Build history of the part. All positions in model axes, mm. A direction names the side the tool comes from. Round coordinates to 2 decimals unless told otherwise and drop trailing zeros. Loops run counter-clockwise (first coordinate to the right, second up) from the corner with the lowest first, then second, coordinate; pieces in that order, holes last. Notation, with made-up numbers: (-1, 26.25) - (19, 26.25) arc R10 cw to (19, 44.25) - close; hole circle Ø8 at (-38, 10). An arc over 180 degrees is marked (long way). Answer as CSV lines item,"result". Start each with the question number.
```python
from build123d import *

# Parameters (mm, degrees)
SKETCH_R      = 54
SKETCH_R_2    = 32
SKETCH_R_3    = 2.5
PAD_DEPTH     = 3
SKETCH001_R   = 37.5
SKETCH001_R_2 = 32.5
PAD001_DEPTH  = 4
SKETCH002_R   = 42
SKETCH002_R_2 = 37.5
PAD002_DEPTH  = 18
SKETCH003_R   = 48
SKETCH003_R_2 = 42
PAD003_DEPTH  = 5
SKETCH004_R   = 32
SKETCH004_R_2 = 5.25
POCKET_DEPTH  = 18.001
CHAMFER_SIZE  = 1


with BuildPart() as part:
    # Sketch → Pad (new body)
    with BuildSketch(Plane.XY):
        Circle(SKETCH_R)
        Circle(SKETCH_R_2, mode=Mode.SUBTRACT)
        with Locations((31.496593, 37.536178)):
            Circle(SKETCH_R_3, mode=Mode.SUBTRACT)
        with Locations((48.25558, 8.508761)):
            Circle(SKETCH_R_3, mode=Mode.SUBTRACT)
        with Locations((42.435245, -24.5)):
            Circle(SKETCH_R_3, mode=Mode.SUBTRACT)
        with Locations((16.758987, -46.044938)):
            Circle(SKETCH_R_3, mode=Mode.SUBTRACT)
        with Locations((-16.758987, -46.044938)):
            Circle(SKETCH_R_3, mode=Mode.SUBTRACT)
        with Locations((-42.435245, -24.5)):
            Circle(SKETCH_R_3, mode=Mode.SUBTRACT)
        with Locations((-48.25558, 8.508761)):
            Circle(SKETCH_R_3, mode=Mode.SUBTRACT)
        with Locations((-31.496593, 37.536178)):
            Circle(SKETCH_R_3, mode=Mode.SUBTRACT)
        with Locations((0, 49)):
            Circle(SKETCH_R_3, mode=Mode.SUBTRACT)
    extrude(amount=PAD_DEPTH)

    # Sketch001 (on Face13 of Pad) → Pad001 (join)
    with BuildSketch(Plane.XY.offset(3)):
        Circle(SKETCH001_R)
        Circle(SKETCH001_R_2, mode=Mode.SUBTRACT)
    extrude(amount=PAD001_DEPTH)

    # Sketch002 (on Face3 of Pad001) → Pad002 (join)
    with BuildSketch(Plane.XY.offset(3)):
        Circle(SKETCH002_R)
        Circle(SKETCH002_R_2, mode=Mode.SUBTRACT)
    extrude(amount=PAD002_DEPTH)

    # Sketch003 (on Face3 of Pad002) → Pad003 (join)
    with BuildSketch(Plane.XY.offset(3)):
        Circle(SKETCH003_R)
        Circle(SKETCH003_R_2, mode=Mode.SUBTRACT)
    extrude(amount=PAD003_DEPTH)

    # Sketch004 → Pocket (cut, through all)
    with BuildSketch(Plane.XY.offset(3)):
        Circle(SKETCH004_R)
        with Locations((31.496593, 37.536178)):
            Circle(SKETCH004_R_2)
        with Locations((48.25558, 8.508761)):
            Circle(SKETCH004_R_2)
        with Locations((42.435245, -24.5)):
            Circle(SKETCH004_R_2)
        with Locations((16.758987, -46.044938)):
            Circle(SKETCH004_R_2)
        with Locations((-16.758987, -46.044938)):
            Circle(SKETCH004_R_2)
        with Locations((-42.435245, -24.5)):
            Circle(SKETCH004_R_2)
        with Locations((-48.25558, 8.508761)):
            Circle(SKETCH004_R_2)
        with Locations((-31.496593, 37.536178)):
            Circle(SKETCH004_R_2)
        with Locations((0, 49)):
            Circle(SKETCH004_R_2)
    extrude(amount=POCKET_DEPTH, mode=Mode.SUBTRACT)

    # Chamfer
    chamfer_edges = [part.edges().sort_by_distance(p)[0] for p in [
        (-37.5, 0, 21),
        (-42, 0, 21),
    ]]
    chamfer(chamfer_edges, length=CHAMFER_SIZE)


solid = part.part
```
Q1. Pin check, flat tips, straight feed: pin 1 Ø5 at (x, y) = (-33, 3.5) entering from -Z; pin 2 Ø2 at (x, y) = (32, 34.5) entering from +Z; pin 3 Ø1.5 at (x, z) = (-19.5, 4.5) entering from +Y; pin 4 Ø8 at (y, z) = (18.5, 17.5) entering from +X. Stop position of each tip, or through.
Q2. Wall check: probe 1 along Y at (x, z) = (0, 16); probe 2 along Z at (x, y) = (-40, 33); probe 3 along Z at (x, y) = (-15, -31). Give the ranges that are in metal, low to high. Write a range as [from, to].
Q3. Band-saw the part on B-B, the plane z = 4.75. List the corners of the cut face in (x, y), then the cut area to 3 significant figures.
Q4. Tool access for faces 4 (the cylindrical face through (31, 9.76, 4.97)), 5 (the cylindrical face through (-16.26, 45.16, 5.46)), 6 (the cylindrical face through (-0.1, 43.75, 5.46)): list every direction of +Z, -Z, +X, -X, +Y, -Y with a clear straight run to the whole face (end or side of a thin tool).
Q5. Band-saw the part on C-C, the plane x = 0. Give the number of separate pieces and of enclosed holes in the cut face, then the cut area to 3 significant figures.
Q6. Band-saw the part on D-D, the plane y = 49. List the corners of the cut face in (x, z).
Q7. Band-saw the part on A-A, the plane y = 0. List the corners of the cut face in (x, z).
Q8. Two-plate mould, pull along X, no slides. Class faces 1 (the cylindrical face through (-47.3, -8.17, 5.46)), 2 (the cylindrical face through (-28.2, 33.45, 5.46)), 3 (the cylindrical face through (41.65, 23.86, 5.46)): released by +X, released by -X, zero draft, split by the parting line, or undercut.
Reported:
1,pin 1,"stops at z = 0"
1,pin 2,"stops at z = 3"
1,pin 3,"stops at y = 44.19"
1,pin 4,"stops at x = 39.42"
2,probe 1,"y = [-42, -37.5], [37.5, 42]"
2,probe 2,"z = [0, 3]"
2,probe 3,"z = [0, 7]"
3,outline,"(-47.89, 3.27) arc R48 ccw to (-43.88, -19.45) arc R5.25 cw to (-38.79, -28.28) arc R48 ccw to (-21.11, -43.11) arc R5.25 cw to (-11.54, -46.59) arc R48 ccw to (11.54, -46.59) arc R5.25 cw to (21.11, -43.11) arc R48 ccw to (38.79, -28.28) arc R5.25 cw to (43.88, -19.45) arc R48 ccw to (47.89, 3.27) arc R5.25 cw to (46.12, 13.3) arc R48 ccw to (34.58, 33.29) arc R5.25 cw to (26.78, 39.84) arc R48 ccw to (5.09, 47.73) arc R5.25 cw to (-5.09, 47.73) arc R48 ccw to (-26.78, 39.84) arc R5.25 cw to (-34.58, 33.29) arc R48 ccw to (-46.12, 13.3) arc R5.25 cw to start; hole circle Ø65 at (0, 0)"
3,area,"3,630 mm2"
4,face 4,"+Z"
4,face 5,"+Z, -X, +Y"
4,face 6,"+Z, +Y"
5,separate pieces,"3"
5,enclosed holes,"0"
5,area,"356 mm2"
6,outline,"(-22.69, 0) - (-2.5, 0) - (-2.5, 3) - (-22.69, 3) - close; (2.5, 0) - (22.69, 0) - (22.69, 3) - (2.5, 3) - close"
7,outline,"(-54, 0) - (-32, 0) - (-32, 3) - (-32.5, 3) - (-32.5, 7) - (-37.5, 7) - (-37.5, 20) - (-38.5, 21) - (-41, 21) - (-42, 20) - (-42, 8) - (-48, 8) - (-48, 3) - (-54, 3) - close; (32, 0) - (54, 0) - (54, 3) - (48, 3) - (48, 8) - (42, 8) - (42, 20) - (41, 21) - (38.5, 21) - (37.5, 20) - (37.5, 7) - (32.5, 7) - (32.5, 3) - (32, 3) - close"
8,face 1,"released by -X"
8,face 2,"undercut"
8,face 3,"released by +X"
